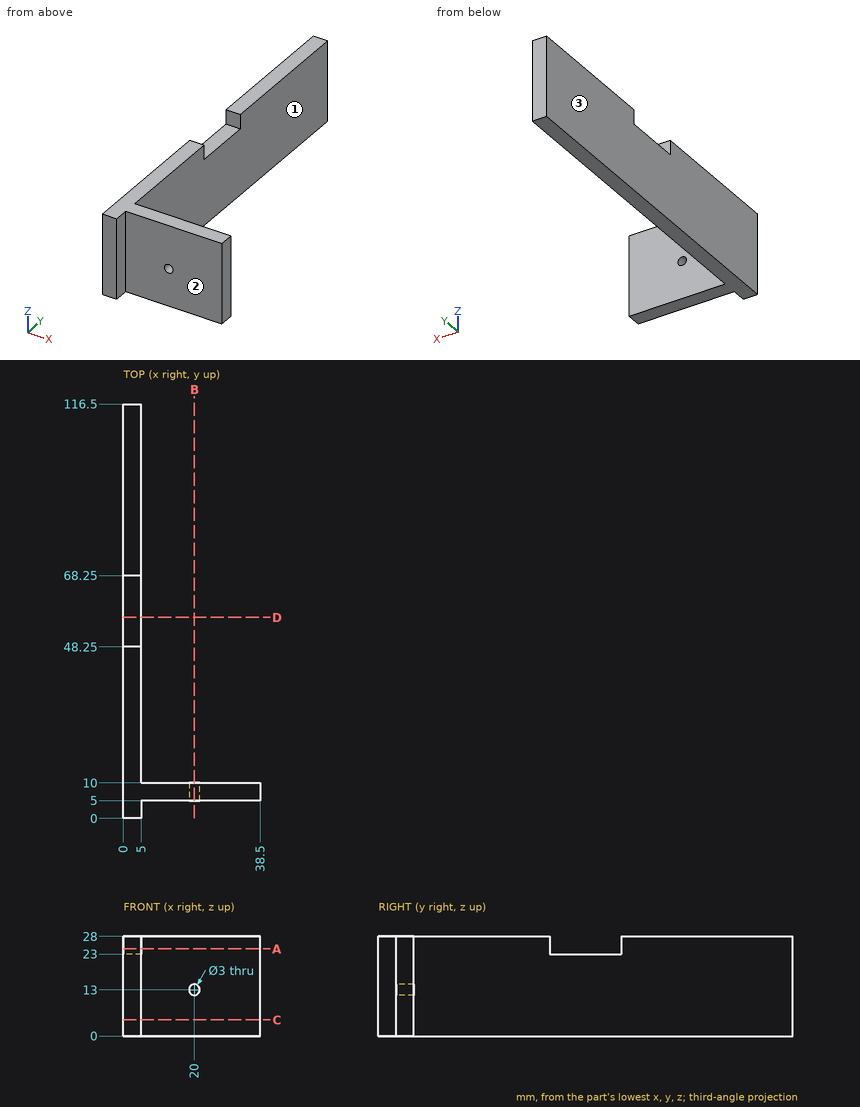
Could you check a few things on this drawing? It's one solid part, dimensions in mm from its lowest x, y, z. A direction names the side the tool comes from. Coordinates: 2 decimals unless noted, no trailing zeros. Write each loop counter-clockwise with the first axis right and the second up, starting at its lowest first coordinate (ties: lowest second). Pieces come first, ordered by that corner, then holes. Notation, with made-up numbers: (-29.75, 10) - (5.25, 10) arc R22 cw to (5.25, 19) - close; hole circle Ø4 at (64.5, 44.25). An arc over 180 degrees is marked (long way). Use one line per item in the form item = value.
1) I'm going to push flat-ended pins straight in: P1, Ø1.5, axis at y = 74.5, z = 4.5, coming from the +X side; P2, Ø8.5, axis at x = 16.5, z = 18, coming from the +Y side; P3, Ø2.5, axis at x = 2, y = 57.5, coming from the +Z side. Where does each tip first touch, or does it pass through?
Solved:
P1 = 5
P2 = 10
P3 = 23
2) Suppose I cut it at C-C, the plane z = 4.5. Write out the boundary of the cut face in (x, y), plus the area to 3 significant figures.
Solved:
outline = (0, 0) - (5, 0) - (5, 5) - (38.5, 5) - (38.5, 10) - (5, 10) - (5, 116.5) - (0, 116.5) - close
area = 750 mm2
3) I need wall thicknesses on line 1 (Z direction, x = 20, y = 6.2); line 2 (Y direction, x = 20, z = 18.25); line 3 (X direction, y = 87, z = 26.25). Which ranges of each line are inside material? Lowest first, please.
Solved:
line_1 = 0 to 11.5, 14.5 to 28
line_2 = 5 to 10
line_3 = 0 to 5
4) Suppose I cut it at D-D, the plane y = 56.5. Write out the boundary of the cut face in (x, z).
Solved:
outline = (0, 0) - (5, 0) - (5, 23) - (0, 23) - close
5) On a 3-axis mill with a long thin cutter (end or side, diameter ignored), from which of +Z, -Z, +X, -X, +Y, -Y can I reach the whole of each face in a straight line? I mean the marked faces 1, 2 and 3. Say none if no direction works.
Solved:
face_1 = +Z, -Z, +X, +Y
face_2 = +Z, -Z, +X, -Y
face_3 = +Z, -Z, -X, +Y, -Y
6) Suppose I cut it at B-B, the plane x = 20. Write out the boundary of the cut face in (y, z), plus the area to 3 significant figures.
Solved:
outline = (5, 0) - (10, 0) - (10, 11.5) - (5, 11.5) - close; (5, 14.5) - (10, 14.5) - (10, 28) - (5, 28) - close
area = 125 mm2
7) Suppose I cut it at A-A, the plane z = 24.5. Write out the boundary of the cut face in (x, y).
Solved:
outline = (0, 0) - (5, 0) - (5, 5) - (38.5, 5) - (38.5, 10) - (5, 10) - (5, 48.25) - (0, 48.25) - close; (0, 68.25) - (5, 68.25) - (5, 116.5) - (0, 116.5) - close
